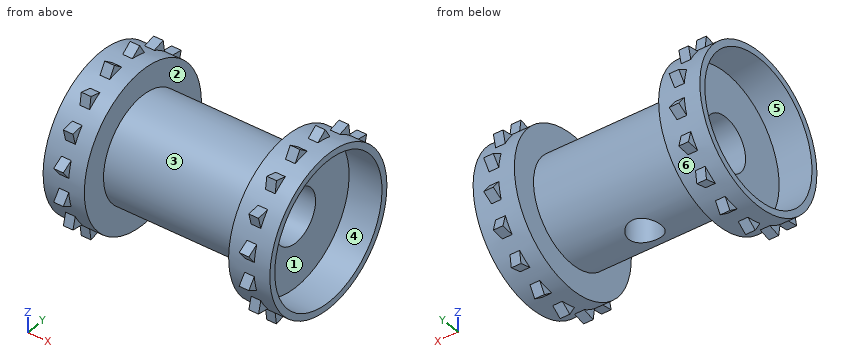
```python
from build123d import *

# Parameters (mm, degrees)
CROQUIS1_R              = 8
CROQUIS1_R_2            = 4.075
SALIENTE_EXTRUIR1_DEPTH = 11.2
CROQUIS3_R              = 11.9
CROQUIS3_R_2            = 4.075
SALIENTE_EXTRUIR2_DEPTH = 1.3
CROQUIS4_R              = 11.9
CROQUIS4_R_2            = 10.9
SALIENTE_EXTRUIR3_DEPTH = 5.1
SALIENTE_EXTRUIR4_DEPTH = 0.75
CROQUIS6_R              = 2.5
CORTAR_EXTRUIR1_DEPTH   = 13.966428038


with BuildPart() as part:
    # Croquis1 → Saliente-Extruir1 (new body, symmetric)
    with BuildSketch(Plane(origin=(0, 0, 0), x_dir=(0, 0, -1), z_dir=(1, 0, 0))):
        Circle(CROQUIS1_R)
        Circle(CROQUIS1_R_2, mode=Mode.SUBTRACT)
    extrude(amount=SALIENTE_EXTRUIR1_DEPTH, both=True)

    # Croquis3 → Saliente-Extruir2 (add)
    with BuildSketch(Plane(origin=(11.2, 0, 0), x_dir=(0, 0, -1), z_dir=(1, 0, 0))):
        Circle(CROQUIS3_R)
        Circle(CROQUIS3_R_2, mode=Mode.SUBTRACT)
    saliente_extruir2 = extrude(amount=SALIENTE_EXTRUIR2_DEPTH)

    # Croquis4 → Saliente-Extruir3 (add)
    with BuildSketch(Plane(origin=(12.5, 0, 0), x_dir=(0, 0, -1), z_dir=(1, 0, 0))):
        Circle(CROQUIS4_R)
        Circle(CROQUIS4_R_2, mode=Mode.SUBTRACT)
    saliente_extruir3 = extrude(amount=SALIENTE_EXTRUIR3_DEPTH)

    # Simetría1: Saliente-Extruir2, Saliente-Extruir3 across plane
    add(saliente_extruir2.mirror(Plane(origin=(0, 0, 0), x_dir=(0, 0, 1), z_dir=(1, 0, 0))))
    add(saliente_extruir3.mirror(Plane(origin=(0, 0, 0), x_dir=(0, 0, 1), z_dir=(1, 0, 0))))

    # Croquis5 → Saliente-Extruir4 (add, symmetric)
    with BuildSketch(Plane(origin=(14.4, 0, 0), x_dir=(0, 0, -1), z_dir=(1, 0, 0))):
        with BuildLine():
            Line((2.579182897, 12.966428038), (3.534712981, 11.362913541))
            ThreePointArc((3.534712981, 11.362913541), (2.321574832, 11.671344837), (1.08274978, 11.850639346))
            Line((1.08274978, 11.850639346), (2.579182897, 12.966428038))
        make_face()
        with BuildLine():
            Line((7.344891477, 10.99240691), (7.614047732, 9.145287155))
            ThreePointArc((7.614047732, 9.145287155), (6.611285773, 9.894488386), (5.535373701, 10.534212737))
            Line((5.535373701, 10.534212737), (7.344891477, 10.99240691))
        make_face()
        with BuildLine():
            Line((10.99240691, 7.344891477), (10.534212737, 5.535373701))
            ThreePointArc((10.534212737, 5.535373701), (9.894488386, 6.611285773), (9.145287155, 7.614047732))
            Line((9.145287155, 7.614047732), (10.99240691, 7.344891477))
        make_face()
        with BuildLine():
            Line((12.966428038, 2.579182897), (11.850639346, 1.08274978))
            ThreePointArc((11.850639346, 1.08274978), (11.671344837, 2.321574832), (11.362913541, 3.534712981))
            Line((11.362913541, 3.534712981), (12.966428038, 2.579182897))
        make_face()
        with BuildLine():
            Line((12.966428038, -2.579182897), (11.362913541, -3.534712981))
            ThreePointArc((11.362913541, -3.534712981), (11.671344837, -2.321574832), (11.850639346, -1.08274978))
            Line((11.850639346, -1.08274978), (12.966428038, -2.579182897))
        make_face()
        with BuildLine():
            Line((10.99240691, -7.344891477), (9.145287155, -7.614047732))
            ThreePointArc((9.145287155, -7.614047732), (9.894488386, -6.611285773), (10.534212737, -5.535373701))
            Line((10.534212737, -5.535373701), (10.99240691, -7.344891477))
        make_face()
        with BuildLine():
            Line((7.344891477, -10.99240691), (5.535373701, -10.534212737))
            ThreePointArc((5.535373701, -10.534212737), (6.611285773, -9.894488386), (7.614047732, -9.145287155))
            Line((7.614047732, -9.145287155), (7.344891477, -10.99240691))
        make_face()
        with BuildLine():
            Line((2.579182897, -12.966428038), (1.08274978, -11.850639346))
            ThreePointArc((1.08274978, -11.850639346), (2.321574832, -11.671344837), (3.534712981, -11.362913541))
            Line((3.534712981, -11.362913541), (2.579182897, -12.966428038))
        make_face()
        with BuildLine():
            Line((-2.579182897, -12.966428038), (-3.534712981, -11.362913541))
            ThreePointArc((-3.534712981, -11.362913541), (-2.321574832, -11.671344837), (-1.08274978, -11.850639346))
            Line((-1.08274978, -11.850639346), (-2.579182897, -12.966428038))
        make_face()
        with BuildLine():
            Line((-7.344891477, -10.99240691), (-7.614047732, -9.145287155))
            ThreePointArc((-7.614047732, -9.145287155), (-6.611285773, -9.894488386), (-5.535373701, -10.534212737))
            Line((-5.535373701, -10.534212737), (-7.344891477, -10.99240691))
        make_face()
        with BuildLine():
            Line((-10.99240691, -7.344891477), (-10.534212737, -5.535373701))
            ThreePointArc((-10.534212737, -5.535373701), (-9.894488386, -6.611285773), (-9.145287155, -7.614047732))
            Line((-9.145287155, -7.614047732), (-10.99240691, -7.344891477))
        make_face()
        with BuildLine():
            Line((-12.966428038, -2.579182897), (-11.850639346, -1.08274978))
            ThreePointArc((-11.850639346, -1.08274978), (-11.671344837, -2.321574832), (-11.362913541, -3.534712981))
            Line((-11.362913541, -3.534712981), (-12.966428038, -2.579182897))
        make_face()
        with BuildLine():
            Line((-12.966428038, 2.579182897), (-11.362913541, 3.534712981))
            ThreePointArc((-11.362913541, 3.534712981), (-11.671344837, 2.321574832), (-11.850639346, 1.08274978))
            Line((-11.850639346, 1.08274978), (-12.966428038, 2.579182897))
        make_face()
        with BuildLine():
            Line((-10.99240691, 7.344891477), (-9.145287155, 7.614047732))
            ThreePointArc((-9.145287155, 7.614047732), (-9.894488386, 6.611285773), (-10.534212737, 5.535373701))
            Line((-10.534212737, 5.535373701), (-10.99240691, 7.344891477))
        make_face()
        with BuildLine():
            Line((-7.344891477, 10.99240691), (-5.535373701, 10.534212737))
            ThreePointArc((-5.535373701, 10.534212737), (-6.611285773, 9.894488386), (-7.614047732, 9.145287155))
            Line((-7.614047732, 9.145287155), (-7.344891477, 10.99240691))
        make_face()
        with BuildLine():
            Line((-2.579182897, 12.966428038), (-1.08274978, 11.850639346))
            ThreePointArc((-1.08274978, 11.850639346), (-2.321574832, 11.671344837), (-3.534712981, 11.362913541))
            Line((-3.534712981, 11.362913541), (-2.579182897, 12.966428038))
        make_face()
    saliente_extruir4 = extrude(amount=SALIENTE_EXTRUIR4_DEPTH, both=True)

    # Simetría2: Saliente-Extruir4 across plane
    add(saliente_extruir4.mirror(Plane(origin=(0, 0, 0), x_dir=(0, 0, 1), z_dir=(1, 0, 0))))

    # Croquis6 → Cortar-Extruir1 (cut, through all)
    with BuildSketch(Plane.XY):
        Circle(CROQUIS6_R)
    extrude(amount=-CORTAR_EXTRUIR1_DEPTH, mode=Mode.SUBTRACT)


solid = part.part
```
For this review, take the finished solid that the model builds, in its own axes (mm). Face numbers are marked on the shaded views. A direction names the side the tool comes from. Give positions to 0.01 mm unless a question says otherwise; leave off trailing zeros. Write each loop counter-clockwise with the first axis right and the second up, starting at its lowest first coordinate (ties: lowest second). Pieces come first, ordered by that corner, then holes. Notation, with made-up numbers: M 86.25,75.25 L 124.25,75.25 A24 cw 124.25,101.25 Z; hole C -5,43.5 d4. An arc over 180 degrees is marked long. Answer as a JSON object with one key per item and string values. Group by question number.
Item 1: Consider section D-D on x = -3. Write out the cut boundary in (y, z) (3 decimals).
Item 2: Draft analysis for pull direction Y (two halves, no side actions). For the marked faces 1, 2 and 3, state which applies: +Y half, -Y half, draft (parallel to the pull), parting line (faces both ways), or undercut.
Item 3: For probe 1 along X at (y, z) = (9.25, 0.5); probe 2 along Y at (x, z) = (-16.4, 0); probe 3 along X at (y, z) = (11, -3.25), list the stretches that pass through material, from the lowest coordinate up. Write a range as [from, to].
Item 4: Consider section B-B on y = 0. Write out the cut boundary in (x, z) (3 decimals).
Item 5: For pin 1 Ø1.8 at (y, z) = (12.5, 3) entering from +X; pin 2 Ø4 at (y, z) = (-5, 4.5) entering from +X; pin 3 Ø0.5 at (y, z) = (12, -2.5) entering from -X; pin 4 Ø1.5 at (x, y) = (7, -10) entering from +Z, all flat-tipped, find the tip position at first contact; note any pin that passes through.
Item 6: Consider section A-A on z = 0. Write out the cut boundary in (x, y) (3 decimals).
Item 7: Tool access review of the marked faces 4, 5 and 6: name each direction out of +Z, -Z, +X, -X, +Y, -Y from which nothing blocks a thin tool from reaching the whole face with its end or side.
Check result:
{
 "1": {"outline": "C 0,0 d16; hole C 0,0 d8.15"},
 "2": {"face 1": "undercut", "face 2": "draft", "face 3": "parting line"},
 "3": {"probe 1": "x = [-12.5, -11.2], [11.2, 12.5]", "probe 2": "y = [-11.9, -10.9], [10.9, 11.9]", "probe 3": "x = [-17.6, -11.2], [11.2, 17.6]"},
 "4": {"outline": "M -17.6,-11.9 L -11.2,-11.9 L -11.2,-8 L -2.5,-8 L -2.5,-4.075 L -12.5,-4.075 L -12.5,-10.9 L -17.6,-10.9 Z; M -17.6,10.9 L -12.5,10.9 L -12.5,4.075 L 12.5,4.075 L 12.5,10.9 L 17.6,10.9 L 17.6,11.9 L 11.2,11.9 L 11.2,8 L -11.2,8 L -11.2,11.9 L -17.6,11.9 Z; M 2.5,-8 L 11.2,-8 L 11.2,-11.9 L 17.6,-11.9 L 17.6,-10.9 L 12.5,-10.9 L 12.5,-4.075 L 2.5,-4.075 Z"},
 "5": {"pin 1": "stops at x = 15.15", "pin 2": "stops at x = 12.5", "pin 3": "stops at x = -15.15", "pin 4": "passes through"},
 "6": {"outline": "M -17.6,-11.9 L -11.2,-11.9 L -11.2,-8 L 11.2,-8 L 11.2,-11.9 L 17.6,-11.9 L 17.6,-10.9 L 12.5,-10.9 L 12.5,-4.075 L -12.5,-4.075 L -12.5,-10.9 L -17.6,-10.9 Z; M -17.6,10.9 L -12.5,10.9 L -12.5,4.075 L 12.5,4.075 L 12.5,10.9 L 17.6,10.9 L 17.6,11.9 L 11.2,11.9 L 11.2,8 L -11.2,8 L -11.2,11.9 L -17.6,11.9 Z"},
 "7": {"face 4": "+X", "face 5": "-X", "face 6": "none"}
}
